Study the drawing (mm; zero at the part's minimum x, y, z) and answer. A direction names the side the tool comes from. Round coordinates to 2 decimals unless told otherwise and drop trailing zeros. Order: outer loops, then holes, each group sorted by start corner. A loop starts at its lowest first (then second) coordinate and runs counter-clockwise, first axis right, second up. Notation, with made-up numbers: (37, 79) -> (74, 79) arc R9 cw to (74, 91) -> close; hole circle Ø2 at (42, 20). An arc over 180 degrees is marked (long way). Use one line per item in the form item = value.
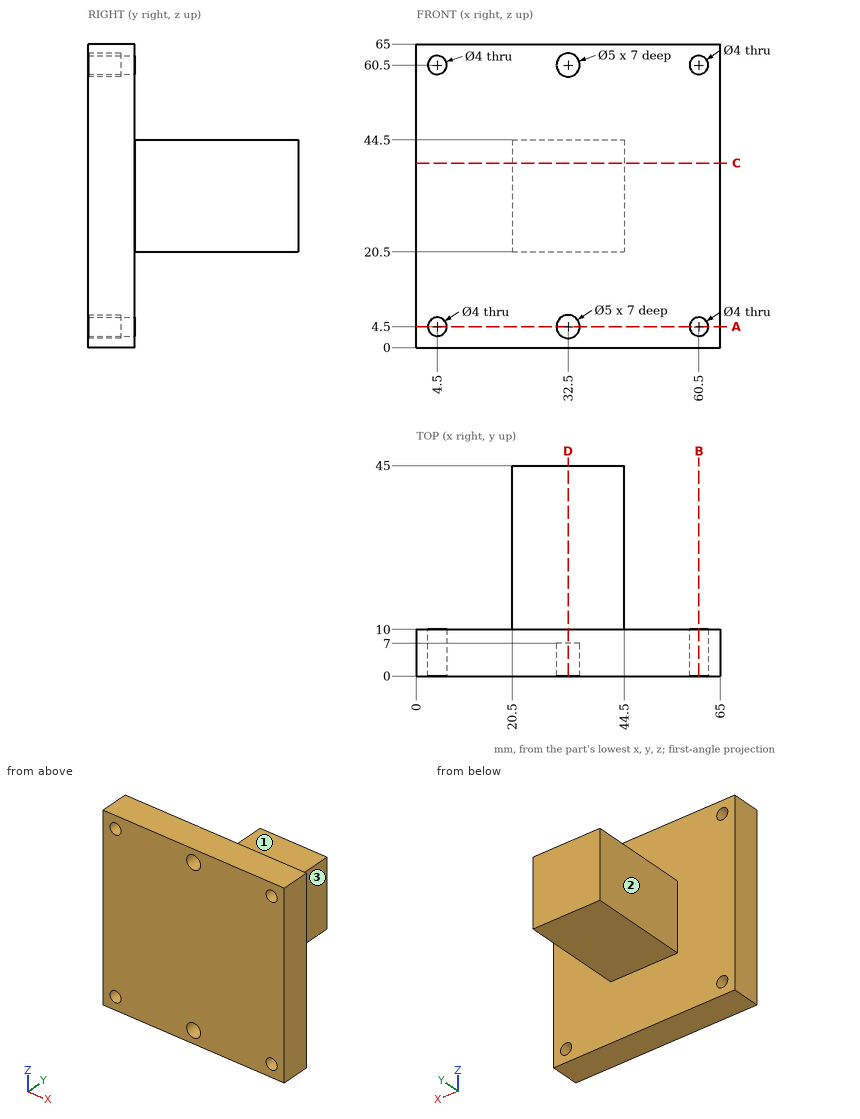
Item 1: The part is cut by section B-B, the plane x = 60.5. Give the vertices of the cut face in (y, z), and give its area (3 significant figures).
Findings:
outline = (0, 0) -> (10, 0) -> (10, 2.5) -> (0, 2.5) -> close; (0, 6.5) -> (10, 6.5) -> (10, 58.5) -> (0, 58.5) -> close; (0, 62.5) -> (10, 62.5) -> (10, 65) -> (0, 65) -> close
area = 570 mm^2
Item 2: The part is cut by section C-C, the plane z = 39.5. Give the vertices of the cut face in (x, y), and give its area (3 significant figures).
Findings:
outline = (0, 0) -> (65, 0) -> (65, 10) -> (44.5, 10) -> (44.5, 45) -> (20.5, 45) -> (20.5, 10) -> (0, 10) -> close
area = 1,490 mm^2
Item 3: Flat-ended cylindrical pins translate along their axes: P1, Ø12, axis at x = 28, y = 27.5, coming from the -Z side; P2, Ø2.5, axis at x = 33, z = 61, coming from the -Y side; P3, Ø3, axis at y = 13, z = 56, coming from the +X side; P4, Ø4.5, axis at x = 60.5, z = 60.5, coming from the +Y side. Find the tip coordinate at first contact, or state that the pin passes through.
Findings:
P1 = 20.5
P2 = 7
P3 = through
P4 = 10
Item 4: For the marked faces 1, 2 and 3, determine the directions among +Z, -Z, +X, -X, +Y, -Y from which every point of the face is accessible in a straight line to the end or side of a thin tool.
Findings:
face_1 = +Z, +X, -X, +Y
face_2 = +Z, -Z, -X, +Y
face_3 = +Z, -Z, +X, +Y
Item 5: The part is cut by section D-D, the plane x = 32.5. Give the vertices of the cut face in (y, z), and give its area (3 significant figures).
Findings:
outline = (0, 0) -> (10, 0) -> (10, 20.5) -> (45, 20.5) -> (45, 44.5) -> (10, 44.5) -> (10, 65) -> (0, 65) -> (0, 63) -> (7, 63) -> (7, 58) -> (0, 58) -> (0, 7) -> (7, 7) -> (7, 2) -> (0, 2) -> close
area = 1,420 mm^2
Item 6: Consider line 1 along Z through (x, y) = (60.5, 7); line 2 along X through (y, z) = (36, 25); line 3 along Y through (x, z) = (28, 3.5). Determine where each line is inside the solid, lowest interval first.
Findings:
line_1 = 0 to 2.5, 6.5 to 58.5, 62.5 to 65
line_2 = 20.5 to 44.5
line_3 = 0 to 10
Item 7: The part is cut by section A-A, the plane z = 4.5. Give the vertices of the cut face in (x, y).
Findings:
outline = (0, 0) -> (2.5, 0) -> (2.5, 10) -> (0, 10) -> close; (6.5, 0) -> (30, 0) -> (30, 7) -> (35, 7) -> (35, 0) -> (58.5, 0) -> (58.5, 10) -> (6.5, 10) -> close; (62.5, 0) -> (65, 0) -> (65, 10) -> (62.5, 10) -> close
